Autodesk Fusion 360 part; units mm, degrees
sketch "Sketch1" plane through (0, 0, 0) normal (0, 0, 1) x (1, 0, 0) in component "Component"
  circle A0 centre (0, 0) radius 3
  circle A1 centre (0, 0) radius 4
  dimension "d1" = 6
  dimension "d2" = 8
extrude "Extrude1" add sketch "Sketch1" along normal blind 3.5 in component "Component"
sketch "Sketch2" plane through (0, 0, 3.5) normal (0, 0, 1) x (-1, 0, 0) in component "Component"
  circle A0 centre (0, 0) radius 3
  circle A1 centre (0, 0) radius 4
  circle A2 centre (0, 0) radius 1.5
  dimension "d5" = 3
extrude "Extrude2" add sketch "Sketch2" along normal blind 2 contours A0 | A1 in component "Component"
sketch "Sketch3" plane through (0, 0, 5.5) normal (0, 0, 1) x (-1, 0, 0) in component "Component"
  circle A0 centre (0, 0) radius 1.5
  circle A1 centre (0, 0) radius 4
sketch "Sketch4" plane through (0, 0, 5.5) normal (0, 0, 1) x (1, 0, 0) in component "Component"
  circle A0 centre (0, 0) radius 5
  dimension "d8" = 10
sketch "Sketch5" plane through (0, 0, 5.5) normal (0, 0, 1) x (1, 0, 0) in component "Component"
sketch "Sketch6" plane through (0, 0, 0) normal (0, 1, 0) x (1, 0, 0) in component "Component"
  line L0 (4, 0) -> (5, -5.5)
  line L1 (4, 0) -> (4, -5.5)
  line L2 (4, -5.5) -> (5, -5.5)
sketch "Sketch7" plane through (0, 0, 5.5) normal (0, 0, 1) x (1, 0, 0) in component "Component"
sketch "Sketch8" plane through (0, 0, 0) normal (0, 1, 0) x (1, 0, 0) in component "Component"
  line L0 (0, -5.5) -> (0, 0)
revolve "Revolve1" add sketch "Sketch6" angle 360 about axis through (0, 0, 5.5) along (0, 0, -1) in component "Component"
fillet "Fillet1" radius 0.5 1 edges at (-4.6616, -1.8081, 5.5) in component "Component"
fillet "Fillet2" radius 0.5 1 edges at (-3.7293, -1.4465, 0) in component "Component"
sketch "Sketch9" plane through (0, 0, 0) normal (0, 1, 0) x (1, 0, 0) in component "Component"
sketch "Sketch10" plane through (0, 0, 0) normal (0, 1, 0) x (1, 0, 0) in component "Component"
  line L0 (4, -2.75) -> (1, -2.75)
component "Component" placed x (1, 0, 0) y (0, 1, 0) z (0, 0, 1) at (0, 0, 0)
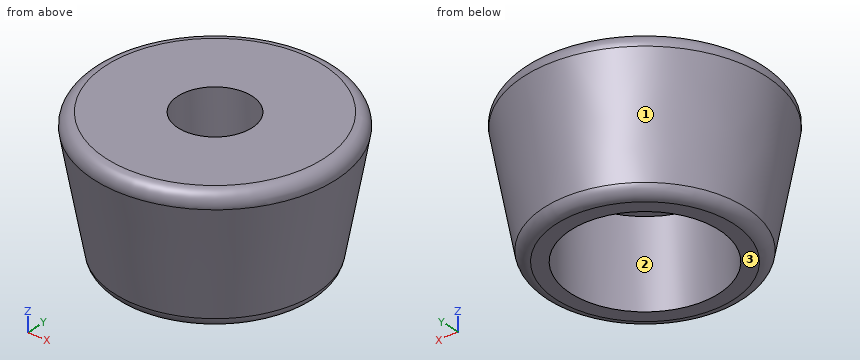
Geometry check sheet. Reference: the model listing, model coordinates, mm. Face numbers are marked on the shaded views. Round coordinates to 2 decimals unless told otherwise and drop trailing zeros. Order: outer loops, then holes, each group sorted by start corner. A loop starts at its lowest first (then second) coordinate and runs counter-clockwise, first axis right, second up. Notation, with made-up numbers: (19.5, 86) -> (44.5, 86) arc R7 cw to (44.5, 90) -> close; hole circle Ø4 at (-24, -9.5). An arc over 180 degrees is marked (long way). Return JSON: item names as keys, results as strings. Group by question number.
Q1. Gauge pin test, flat ends, axial feed: pin 1 (3 mm diameter, centred on x = -4, z = 4.5, fed in from -Y); pin 2 (2 mm diameter, centred on y = -2.5, z = 1.5, fed in from +X). Record the tip position at first contact, or that the pin passes through.
Q2. Release check for a two-part mould opening along X. For the marked faces 1, 2 and 3 record: released by +X, released by -X, zero draft, split by the parting line, or undercut.
Q3. Section check C-C, the plane z = 0.6. Record the boundary of the cut face in (x, y).
Q4. Section check D-D, the plane z = 5.05. Record the boundary of the cut face in (x, y).
Q5. Section check A-A, the plane y = 0. Record the boundary of the cut face in (x, z), plus the area to 3 significant figures.
Q6. Material ranges on probe 1 along X at (y, z) = (0, 4.9); probe 2 along Z at (x, y) = (1.5, 1.75), recorded low to high. Write a range as from..to.
Numbers:
{
 "1": {"pin 1": "y = -4.17", "pin 2": "x = 4.05"},
 "2": {"face 1": "split by the parting line", "face 2": "undercut", "face 3": "zero draft"},
 "3": {"outline": "circle Ø8.22 at (0, 0); hole circle Ø6 at (0, 0)"},
 "4": {"outline": "circle Ø9.8 at (0, 0); hole circle Ø3 at (0, 0)"},
 "5": {"outline": "(-4.89, 4.91) -> (-4.07, 0.41) arc R0.5 ccw to (-3.58, 0) -> (-3, 0) -> (-3, 3.5) -> (-1.5, 3.5) -> (-1.5, 5.5) -> (-4.4, 5.5) arc R0.5 ccw to start; (1.5, 3.5) -> (3, 3.5) -> (3, 0) -> (3.58, 0) arc R0.5 ccw to (4.07, 0.41) -> (4.89, 4.91) arc R0.5 ccw to (4.4, 5.5) -> (1.5, 5.5) -> close", "area": "22.3 mm^2"},
 "6": {"probe 1": "-4.89..-1.5, 1.5..4.89", "probe 2": "3.5..5.5"}
}
